The listing builds one solid part. Answer for the finished solid, in the listing's coordinates (mm). A direction names the side the tool comes from. Coordinates: 2 decimals unless noted, no trailing zeros. Loops run counter-clockwise (first coordinate to the right, second up) from the corner with the lowest first, then second, coordinate; pieces in that order, holes last. Notation, with made-up numbers: (-7.5, 10) - (46.5, 10) arc R32 ccw to (46.5, 45) - close; hole circle Ø10 at (84.5, 70). An arc over 180 degrees is marked (long way). One line per question, with ' | ' between items.
from build123d import *

# Parameters (mm, degrees)
F0_W     = 33
F0_H     = 21
F0_W_2   = 15
F0_H_2   = 15
F0_W_3   = 11
F0_H_3   = 11
F1_DEPTH = 2
F2_DEPTH = 17
F3_W     = 30
F3_H     = 21
F3_W_2   = 15
F3_H_2   = 15
F3_W_3   = 11
F3_H_3   = 11
F4_DEPTH = 2
F6_DEPTH = 25


with BuildPart() as f1:
    # F0 (on Top) → F1 (new body)
    with BuildSketch(Plane.XY):
        Rectangle(F0_W, F0_H)
        Rectangle(F0_W_2, F0_H_2, mode=Mode.SUBTRACT)
        Rectangle(F0_W_2, F0_H_2)
        Rectangle(F0_W_3, F0_H_3, mode=Mode.SUBTRACT)
    extrude(amount=F1_DEPTH)

    # F0 (on Top) → F2 (join)
    with BuildSketch(Plane.XY):
        Rectangle(F0_W_2, F0_H_2)
        Rectangle(F0_W_3, F0_H_3, mode=Mode.SUBTRACT)
    extrude(amount=F2_DEPTH)

    # F3 (on face) → F4 (join)
    with BuildSketch(Plane.XY.offset(17)):
        Rectangle(F3_W, F3_H)
        Rectangle(F3_W_2, F3_H_2, mode=Mode.SUBTRACT)
        Rectangle(F3_W_2, F3_H_2)
        Rectangle(F3_W_3, F3_H_3, mode=Mode.SUBTRACT)
    extrude(amount=F4_DEPTH)

    # F5 (on face) → F6 (cut)
    with BuildSketch(Plane.XZ.offset(10.5)):
        Polygon((-15.671573, 0), (-16.5, 2), (-16.5, 0), align=None)
        Polygon((16.5, 0), (16.5, 2), (15.671573, 0), align=None)
    extrude(amount=-F6_DEPTH, mode=Mode.SUBTRACT)


solid = f1.part
Item 1: Find section D-D, the plane y = 1.25. Write down the section's boundary in (x, z), plus the area to 3 significant figures.
Taken from the geometry:
outline: (-16.5, 2) - (-15.67, 0) - (-5.5, 0) - (-5.5, 19) - (-15, 19) - (-15, 17) - (-7.5, 17) - (-7.5, 2) - close; (5.5, 0) - (15.67, 0) - (16.5, 2) - (7.5, 2) - (7.5, 17) - (15, 17) - (15, 19) - (5.5, 19) - close | area: 140 mm2
Item 2: Find section B-B, the plane x = -5. Write down the section's boundary in (y, z), plus the area to 3 significant figures.
Taken from the geometry:
outline: (-10.5, 0) - (-5.5, 0) - (-5.5, 19) - (-10.5, 19) - (-10.5, 17) - (-7.5, 17) - (-7.5, 2) - (-10.5, 2) - close; (5.5, 0) - (10.5, 0) - (10.5, 2) - (7.5, 2) - (7.5, 17) - (10.5, 17) - (10.5, 19) - (5.5, 19) - close | area: 100 mm2
Item 3: Find section C-C, the plane z = 4.75. Write down the section's boundary in (x, y).
Taken from the geometry:
outline: (-7.5, -7.5) - (7.5, -7.5) - (7.5, 7.5) - (-7.5, 7.5) - close; hole (-5.5, -5.5) - (5.5, -5.5) - (5.5, 5.5) - (-5.5, 5.5) - close
Item 4: Each of these flat-tipped pins is pushed along its axis until it touches: pin 1 Ø5 at (y, z) = (1, 10) entering from +X; pin 2 Ø9 at (x, z) = (-2, 7.5) entering from +Y; pin 3 Ø1.6 at (y, z) = (-2.5, 18) entering from -X; pin 4 Ø1 at (x, z) = (12, 3) entering from +Y. Where does it stop, or does it pass through?
Taken from the geometry:
pin 1: stops at x = 7.5 | pin 2: stops at y = 7.5 | pin 3: stops at x = -15 | pin 4: passes through
Item 5: Find the intervals of material crossed by line 1 (X direction, y = -2, z = 4.75); line 2 (Z direction, x = 10, y = -4.75); line 3 (Y direction, x = -2, z = 17.5), in increasing order. Write a range as [from, to].
Taken from the geometry:
line 1: x = [-7.5, -5.5], [5.5, 7.5] | line 2: z = [0, 2], [17, 19] | line 3: y = [-10.5, -5.5], [5.5, 10.5]
Item 6: Which of the six approach directions +Z, -Z, +X, -X, +Y, -Y give full straight-line access (tool end or side, diameter ignored) to faces 5 (the face through (0, -7.5, 9)), 6 (the face through (-7.5, 0, 9)), 7 (the face through (15, 0, 18))?
Taken from the geometry:
face 5: +X, -X, -Y | face 6: -X, +Y, -Y | face 7: +Z, +X, +Y, -Y
Item 7: Find section A-A, the plane y = 8.75. Write down the section's boundary in (x, z), plus the area to 3 significant figures.
Taken from the geometry:
outline: (-16.5, 2) - (-15.67, 0) - (15.67, 0) - (16.5, 2) - close; (-15, 17) - (15, 17) - (15, 19) - (-15, 19) - close | area: 124 mm2
Item 8: The mould has two halves that part along Y. Classify faces 1 (the face through (0, -10.5, 18)), 2 (the face through (-8, 0, 2)), 3 (the face through (0, 10.5, 18)), 4 (the face through (-5.5, 0, 9)): pulls with the +Y half, pulls with the -Y half, needs draft (parallel to the pull), parting line crosses it, or undercut.
Taken from the geometry:
face 1: pulls with the -Y half | face 2: needs draft | face 3: pulls with the +Y half | face 4: undercut
